from build123d import *

# Parameters (mm, degrees)
SKETCH_W        = 70.5
SKETCH_H        = 47.97
PAD_DEPTH       = 9.5
THICKNESS_T     = 2.5
PAD001_DEPTH    = 2.5
SKETCH003_R     = 3
POCKET001_DEPTH = 5
SKETCH002_W     = 14
SKETCH002_H     = 7.5
POCKET_DEPTH    = 2.5


with BuildPart() as part:
    # Sketch → Pad (new body)
    with BuildSketch(Plane.XY):
        Rectangle(SKETCH_W, SKETCH_H)
    extrude(amount=PAD_DEPTH)

    # Thickness
    thickness_openings = [part.faces().sort_by_distance(p)[0] for p in [
        (0, 0, 9.5),
        (0, 0, 0),
    ]]
    offset(amount=THICKNESS_T, openings=thickness_openings, kind=Kind.INTERSECTION)

    # Sketch001 → Pad001 (join)
    with BuildSketch(Plane.XY):
        with BuildLine():
            Line((-40.25, 26.5), (-40.25, -26.5))
            ThreePointArc((-40.25, -26.5), (-39.517767, -28.267767), (-37.75, -29))
            Line((-37.75, -29), (40.25, -29))
            Line((40.25, -29), (44.25, -29))
            Line((44.25, -22.65), (44.25, -29))
            Line((44.25, -22.65), (40.25, -24.959401))
            Line((40.25, -14.213533), (40.25, -24.959401))
            Line((44.25, -16.522934), (40.25, -14.213533))
            Line((44.25, -5.777066), (44.25, -16.522934))
            Line((44.25, -5.777066), (40.25, -8.086467))
            Line((40.25, 2.659401), (40.25, -8.086467))
            Line((44.25, 0.35), (40.25, 2.659401))
            Line((44.25, 6.7), (44.25, 0.35))
            Line((42.75, 6.7), (44.25, 6.7))
            ThreePointArc((40.25, 9.2), (40.982233, 7.432233), (42.75, 6.7))
            Line((40.25, 9.2), (40.25, 26.5))
            ThreePointArc((40.25, 26.5), (39.517767, 28.267767), (37.75, 29))
            Line((37.75, 29), (-37.75, 29))
            ThreePointArc((-37.75, 29), (-39.517767, 28.267767), (-40.25, 26.5))
        make_face()
    extrude(amount=-PAD001_DEPTH)

    # Sketch003 (on Face10 of Pad001) → Pocket001 (cut)
    with BuildSketch(Plane.YZ.offset(37.75)):
        with Locations((-0.5, 4.75)):
            Circle(SKETCH003_R)
    extrude(amount=-POCKET001_DEPTH, mode=Mode.SUBTRACT)

    # Sketch002 (on Face7 of Pad001) → Pocket (cut)
    with BuildSketch(Plane(origin=(0, 26.485, 0), x_dir=(-1, 0, 0), z_dir=(0, 1, 0))):
        with Locations((-4.45, 5.75)):
            Rectangle(SKETCH002_W, SKETCH002_H)
    extrude(amount=-POCKET_DEPTH, mode=Mode.SUBTRACT)


solid = part.part
Geometry check sheet. Reference: the model listing, model coordinates, mm. A direction names the side the tool comes from. Round coordinates to 2 decimals unless told otherwise and drop trailing zeros. Loops run counter-clockwise (first coordinate to the right, second up) from the corner with the lowest first, then second, coordinate; pieces in that order, holes last. Notation, with made-up numbers: (-28.5, -2) - (8.5, -2) arc R13 cw to (8.5, 22) - close; hole circle Ø9 at (59.25, 67.5). An arc over 180 degrees is marked (long way). One line per question, with ' | ' between items. Start each with the question number.
1. Tool access check on faces 5 (the face through (0, 0, 0)), 6 (the face through (-2.55, 25, 6)), 7 (the face through (40.25, 18, -1)), 8 (the face through (42.278, -6.916, -1.232)). Record the directions out of +Z, -Z, +X, -X, +Y, -Y that give a thin tool (end or side, any length) a straight path to the whole face; none if there is none.
2. Draft check along Y on faces 1 (the face through (-39.537, -28.248, -1.232)), 2 (the face through (5, 25, 2)), 3 (the face through (39.537, 28.248, -1.232)), 4 (the face through (0, -23.985, 5)). Enter one of: released by +Y, released by -Y, zero draft, split by the parting line, or undercut.
3. Cross-section at C-C on x = 1. Record the cut outline in (y, z) (3 decimals), then the cut area to 3 significant figures.
4. Cross-section at D-D on y = 11.5. Record the cut outline in (x, z).
5. Scan lines: line 1 (X direction, y = -4.5, z = 1.5); line 2 (Y direction, x = 33, z = 6.75) (3 decimals); line 3 (X direction, y = 24.5, z = 2.5). Record each from-to range of solid material in increasing order. Write a range as [from, to].
6. Cross-section at A-A on y = -0.5. Record the cut outline in (x, z), then the cut area to 3 significant figures.
7. Cross-section at B-B on z = 4.75. Record the cut outline in (x, y) (3 decimals), then the cut area to 3 significant figures.
8. Depth check by flat-ended pin: pin 1 (1.2 mm diameter, centred on y = -19.5, z = -1.5, fed in from +X); pin 2 (5.5 mm diameter, centred on y = -0.5, z = 4.75, fed in from -X); pin 3 (3 mm diameter, centred on y = 25, z = 5, fed in from +X). Enter the tip coordinate at first touch or a pass-through.
Taken from the geometry:
1) face 5: +Z | face 6: +Z, +Y | face 7: +Z, -Z, +X, +Y | face 8: +Z, -Z
2) face 1: released by -Y | face 2: zero draft | face 3: released by +Y | face 4: undercut
3) outline: (-29, -2.5) - (29, -2.5) - (29, 0) - (26.485, 0) - (26.485, 2) - (23.985, 2) - (23.985, 0) - (-23.985, 0) - (-23.985, 9.5) - (-26.485, 9.5) - (-26.485, 0) - (-29, 0) - close | area: 174 mm²
4) outline: (-40.25, -2.5) - (40.25, -2.5) - (40.25, 0) - (37.75, 0) - (37.75, 9.5) - (35.25, 9.5) - (35.25, 0) - (-35.25, 0) - (-35.25, 9.5) - (-37.75, 9.5) - (-37.75, 0) - (-40.25, 0) - close
5) line 1: [-37.75, -35.25], [35.25, 37.75] | line 2: [-26.485, -23.985], [23.985, 26.485] | line 3: [-37.75, -2.55], [11.45, 37.75]
6) outline: (-40.25, -2.5) - (40.25, -2.5) - (40.25, 0) - (37.75, 0) - (37.75, 1.75) - (35.25, 1.75) - (35.25, 0) - (-35.25, 0) - (-35.25, 9.5) - (-37.75, 9.5) - (-37.75, 0) - (-40.25, 0) - close; (35.25, 7.75) - (37.75, 7.75) - (37.75, 9.5) - (35.25, 9.5) - close | area: 234 mm²
7) outline: (-37.75, -26.485) - (37.75, -26.485) - (37.75, -3.5) - (35.25, -3.5) - (35.25, -23.985) - (-35.25, -23.985) - (-35.25, 23.985) - (-2.55, 23.985) - (-2.55, 26.485) - (-37.75, 26.485) - close; (11.45, 23.985) - (35.25, 23.985) - (35.25, 2.5) - (37.75, 2.5) - (37.75, 26.485) - (11.45, 26.485) - close | area: 567 mm²
8) pin 1: x = 40.25 | pin 2: x = -37.75 | pin 3: x = 37.75
